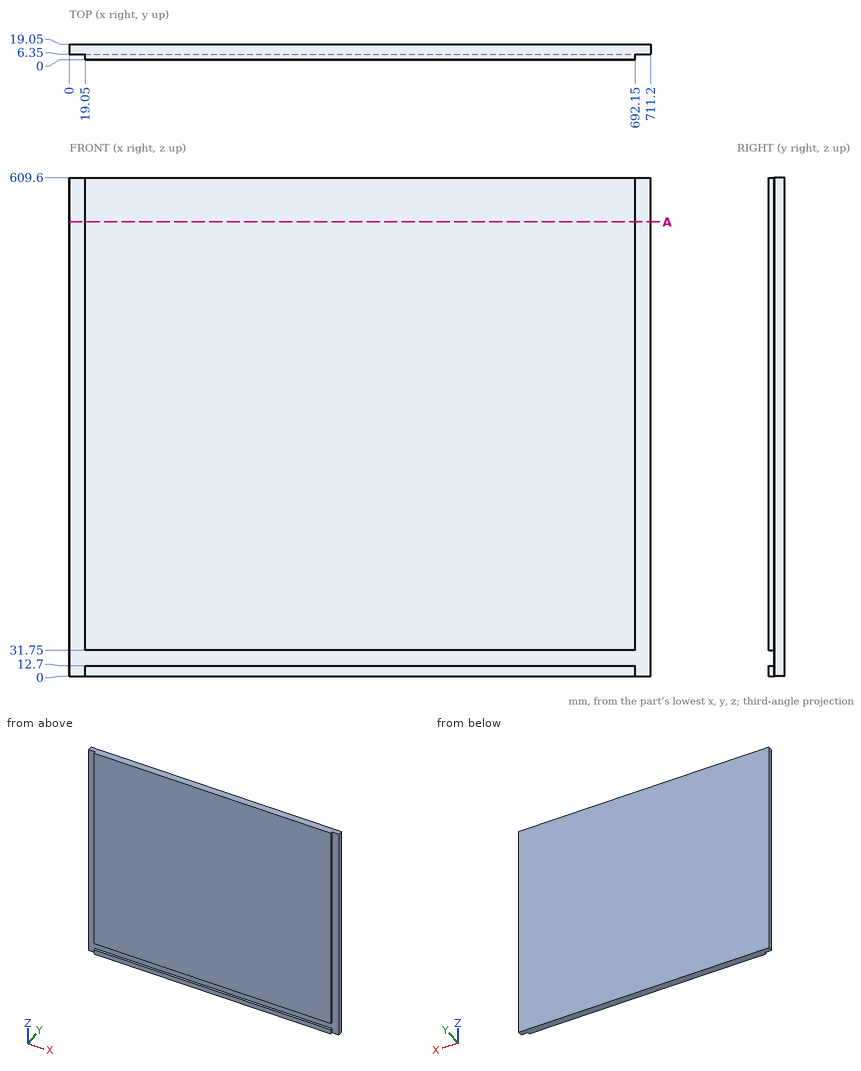
Check sheet for the drawn part. Datum: minimum x, y, z corner. Units: mm. Coordinates: 2 decimals unless noted, no trailing zeros. Order: outer loops, then holes, each group sorted by start corner. A loop starts at its lowest first (then second) coordinate and runs counter-clockwise, first axis right, second up. Notation, with made-up numbers: (47, 37.5) - (95, 37.5) arc R8 ccw to (95, 49.5) - close; hole circle Ø6 at (66.25, -7). An arc over 180 degrees is marked (long way). Return JSON: item names as keys, results as strings.
(1) Thickness scan on line 1 along Z through (x, y) = (656.5, 1.5); line 2 along X through (y, z) = (1.5, 387). Record the ranges inside material, lowest first.
Filled sheet:
{"line 1": "z = 0 to 12.7, 31.75 to 609.6", "line 2": "x = 19.05 to 692.15"}
(2) Section check A-A, the plane z = 555.5. Record the cut outline in (x, y).
Filled sheet:
{"outline": "(0, 6.35) - (19.05, 6.35) - (19.05, 0) - (692.15, 0) - (692.15, 6.35) - (711.2, 6.35) - (711.2, 19.05) - (0, 19.05) - close"}
(3) Go/stop test with flat-tipped pins: pin 1 (1.9 mm diameter, centred on y = 3, z = 344.5, fed in from -X); pin 2 (3 mm diameter, centred on x = 259.5, y = 2.5, fed in from -Z); pin 3 (1.9 mm diameter, centred on y = 4.5, z = 275.5, fed in from +X). Record where each tip stops, or that it passes through.
Filled sheet:
{"pin 1": "stops at x = 19.05", "pin 2": "stops at z = 0", "pin 3": "stops at x = 692.15"}
